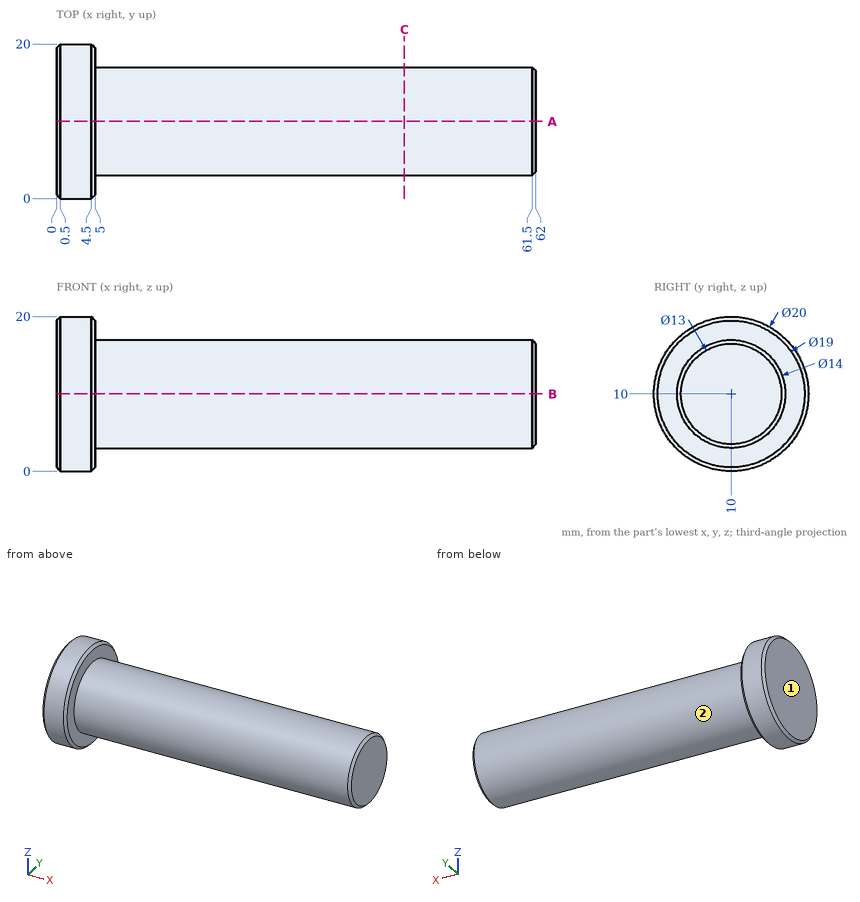
Could you check a few things on this drawing? It's one solid part, dimensions in mm from its lowest x, y, z. A direction names the side the tool comes from. Coordinates: 2 decimals unless noted, no trailing zeros. Write each loop counter-clockwise with the first axis right and the second up, starting at its lowest first coordinate (ties: lowest second). Pieces come first, ordered by that corner, then holes.
1) I'm going to push flat-ended pins straight in: pin 1 (1 mm diameter, centred on x = 35.5, y = 7.5, fed in from +Z); pin 2 (3 mm diameter, centred on x = 51, y = 15.5, fed in from +Z); pin 3 (4 mm diameter, centred on x = 30.5, y = 10.5, fed in from +Z). Where does each tip first touch, or does it pass through?
Filled in:
pin 1: stops at z = 16.71
pin 2: stops at z = 15.74
pin 3: stops at z = 17
2) If we section it at C-C (x = 45): List the corners of the cut face in (y, z) for me, plus the area to 3 significant figures.
Filled in:
outline: circle Ø14 at (10, 10)
area: 154 mm2
3) If I drill on line 1 (X direction, y = 6.75, z = 3.75); line 2 (Y direction, x = 47, z = 5.5); line 3 (Y direction, x = 39, z = 10.5), over which ranges is the centre line in solid material (lowest first)?
Filled in:
line 1: x = 0 to 5
line 2: y = 4.64 to 15.36
line 3: y = 3.02 to 16.98
4) If we section it at A-A (y = 10): List the corners of the cut face in (x, z) for me.
Filled in:
outline: (0, 0.5) - (0.5, 0) - (4.5, 0) - (5, 0.5) - (5, 3) - (61.5, 3) - (62, 3.5) - (62, 16.5) - (61.5, 17) - (5, 17) - (5, 19.5) - (4.5, 20) - (0.5, 20) - (0, 19.5) - close
5) Which directions (+Z, -Z, +X, -X, +Y, -Y) give clear straight access to the entire face, cutting with the end or side of a thin tool? Please do the marked faces 1 and 2.
Filled in:
face 1: +Z, -Z, -X, +Y, -Y
face 2: +X
